Read the model definition and answer for the solid it produces. Units are mm, in the model's axes. Face numbers are marked on the shaded views. A direction names the side the tool comes from. Coordinates: 2 decimals unless noted, no trailing zeros. Write each loop counter-clockwise with the first axis right and the second up, starting at its lowest first coordinate (ties: lowest second). Pieces come first, ordered by that corner, then holes. Notation, with made-up numbers: (-29.5, 32.25) -> (12.5, 32.25) arc R27 ccw to (12.5, 49.25) -> close; hole circle Ø4 at (76, 9.5). An arc over 180 degrees is marked (long way). Return JSON: item names as keys, results as strings.
from build123d import *

# Parameters (mm, degrees)
BOSS_EXTRUDE1_DEPTH = 25.05
SKETCH3_R           = 1.75
CUT_EXTRUDE2_DEPTH  = 35.224258664
FILLET1_R           = 3
BOSS_EXTRUDE2_DEPTH = 15


with BuildPart() as part:
    # Sketch1 → Boss-Extrude1 (new body)
    with BuildSketch(Plane.XY):
        Polygon((0, 0), (-10.247967278, -17.75), (4.876016361, -17.75), (4.876016361, -6), (15, -6), (15, 0), align=None)
    extrude(amount=BOSS_EXTRUDE1_DEPTH)

    # Sketch3 → Cut-Extrude2 (cut, through all)
    with BuildSketch(Plane(origin=(4.876016361, 0, 0), x_dir=(0, 0, -1), z_dir=(1, 0, 0))):
        with Locations(Location((-18.775, -13, 0), (0, 0, 90))):
            Circle(SKETCH3_R)
        with Locations(Location((-6.275, -13, 0), (0, 0, 90))):
            Circle(SKETCH3_R)
    extrude(amount=-CUT_EXTRUDE2_DEPTH, mode=Mode.SUBTRACT)

    # Fillet1
    fillet1_edges = [part.edges().sort_by_distance(p)[0] for p in [
        (4.876016361, -6, 12.525),
    ]]
    fillet(fillet1_edges, radius=FILLET1_R)

    # Sketch4 → Boss-Extrude2 (add)
    with BuildSketch(Plane(origin=(15, 0, 0), x_dir=(0, 0, -1), z_dir=(1, 0, 0))):
        Polygon((-25.05, 8.282359313), (-53.183639918, 36.415999231), (-46.678257531, 42.921381618), (-40.314296501, 36.557420587), (-42.435616844, 34.436100244), (-46.678257531, 38.678740931), (-48.940999231, 36.415999231), (-12.525, 0), (23.890999231, 36.415999231), (21.628257531, 38.678740931), (17.385616844, 34.436100244), (15.264296501, 36.557420587), (21.628257531, 42.921381618), (28.133639918, 36.415999231), (0, 8.282359313), (0, -6), (-25.05, -6), align=None)
    extrude(amount=-BOSS_EXTRUDE2_DEPTH)


solid = part.part
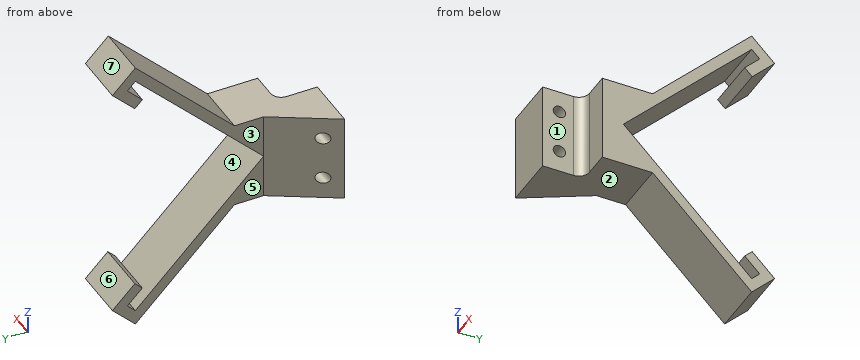
1. The part is cut by section A-A (y = 13). Determine the outline of the cut face in (x, z) (3 decimals).
Taken from the geometry:
{"outline": "(0, -4.718) -> (15, -4.718) -> (15, -0.475) -> (0, -0.475) -> close; (0, 25.525) -> (15, 25.525) -> (15, 29.768) -> (0, 29.768) -> close"}
2. The part is cut by section B-B (x = 12). Determine the outline of the cut face in (y, z) (3 decimals), then the cut area to 3 significant figures.
Taken from the geometry:
{"outline": "(-6, 0) -> (8.282, 0) -> (36.416, -28.134) -> (42.921, -21.628) -> (36.557, -15.264) -> (34.436, -17.386) -> (38.679, -21.628) -> (36.416, -23.891) -> (0, 12.525) -> (36.416, 48.941) -> (38.679, 46.678) -> (34.436, 42.436) -> (36.557, 40.314) -> (42.921, 46.678) -> (36.416, 53.184) -> (8.282, 25.05) -> (-6, 25.05) -> close", "area": "610 mm2"}
3. For a pull along Z with two mould halves and no side action, classify the marked faces 5, 6 and 7 as +Z half, -Z half, draft (parallel to the pull), parting line (faces both ways), or undercut.
Taken from the geometry:
{"face 5": "draft", "face 6": "undercut", "face 7": "+Z half"}
4. Flat-ended cylindrical pins translate along their axes: pin 1 Ø2 at (y, z) = (-13, 18.775) entering from +X; pin 2 Ø4.5 at (y, z) = (-12.5, 6.5) entering from +X; pin 3 Ø2 at (x, z) = (13, 6.5) entering from -Y; pin 4 Ø3 at (x, z) = (-5.5, 16) entering from +Y. Find the tip coordinate at first contact, or state that the pin passes through.
Taken from the geometry:
{"pin 1": "passes through", "pin 2": "stops at x = 4.88", "pin 3": "stops at y = -6", "pin 4": "stops at y = -6.93"}
5. Consider L1, parallel to Z at x = 2, y = -13 (3 decimals); L2, parallel to Z at x = -2, y = -14; L3, parallel to Y at x = -4.25, z = 5. Determine where each line is inside the solid, lowest interval first.
Taken from the geometry:
{"L1": "z = 0 to 4.525, 8.025 to 17.025, 20.525 to 25.05", "L2": "z = 0 to 4.84, 7.71 to 17.34, 20.21 to 25.05", "L3": "y = -17.75 to -14.2, -11.8 to -7.36"}
6. The part is cut by section D-D (z = 15). Determine the outline of the cut face in (x, y) (3 decimals).
Taken from the geometry:
{"outline": "(-10.248, -17.75) -> (4.876, -17.75) -> (4.876, -9) arc R3 cw to (7.876, -6) -> (15, -6) -> (15, 2.475) -> (0, 2.475) -> (0, 0) -> close"}
7. A tool of negligible diameter and unlimited length cuts with its end or side. For the marked faces 1, 2, 3 and 4, from which of +Z, -Z, +X, -X, +Y, -Y can it reach the whole face along a straight path? Write none if from no direction.
Taken from the geometry:
{"face 1": "+Z, -Z, +X, -Y", "face 2": "-Z, +X, -X, -Y", "face 3": "+Z, -Z, -X, +Y", "face 4": "+X, -X"}
8. The part is cut by section C-C (y = -13). Determine the outline of the cut face in (x, z) (3 decimals).
Taken from the geometry:
{"outline": "(-7.506, 0) -> (4.876, 0) -> (4.876, 4.525) -> (-7.506, 4.525) -> close; (-7.506, 8.025) -> (4.876, 8.025) -> (4.876, 17.025) -> (-7.506, 17.025) -> close; (-7.506, 20.525) -> (4.876, 20.525) -> (4.876, 25.05) -> (-7.506, 25.05) -> close"}
